Geometry: final body of the model. Coordinates: model frame, mm. Face numbers are marked on the shaded views. A direction names the side the tool comes from. Give positions to 0.01 mm unless a question says otherwise; leave off trailing zeros. Order: outer loops, then holes, each group sorted by start corner. A loop starts at its lowest first (then second) coordinate and runs counter-clockwise, first axis right, second up. Notation, with made-up numbers: (48, 23.25) - (86, 23.25) arc R23 cw to (86, 61.25) - close; hole circle Ø11 at (82, 4.5). An arc over 180 degrees is marked (long way). Use one line per item in the form item = value.
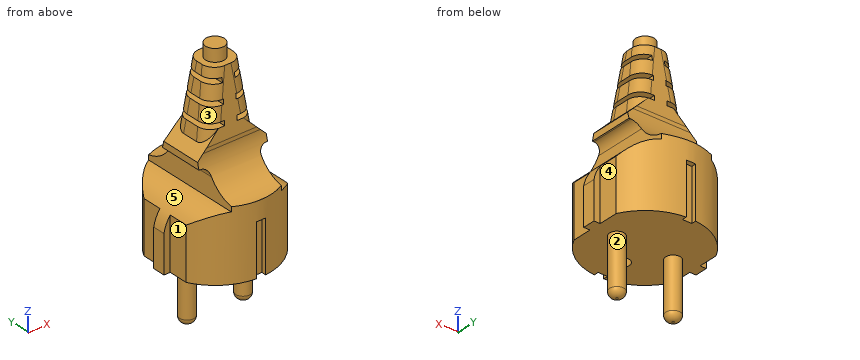
from build123d import *

# Parameters (mm, degrees)
BOSS_EXTRUDE1_DEPTH  = 55.5
SKETCH4_OUTSIDE_W    = 53.062
SKETCH4_OUTSIDE_H    = 72.562
CUT_EXTRUDE3_DEPTH   = 20
CUT_EXTRUDE4_DEPTH   = 16.5
SKETCH6_R            = 5
BOSS_EXTRUDE3_DEPTH  = 55.5
SKETCH7_OUTSIDE_W    = 72.562
SKETCH7_OUTSIDE_H    = 53.062
CUT_EXTRUDE6_DEPTH   = 27.75
FILLET3_R            = 4
SKETCH8_R            = 2.35
BOSS_EXTRUDE4_DEPTH  = 18
FILLET4_R            = 2
FILLET4_OF_MIRROR2_R = 2
SKETCH10_W           = 8.464758564
SKETCH10_H           = 1.5
CUT_EXTRUDE8_DEPTH   = 12
SKETCH11_R           = 3
BOSS_EXTRUDE6_DEPTH  = 59.5
SKETCH12_R           = 2.35
CUT_EXTRUDE9_DEPTH   = 10


with BuildPart() as part:
    # Sketch1 → Boss-Extrude1 (new body)
    with BuildSketch(Plane.XY):
        with BuildLine():
            Line((-16, 2), (-16, 8.246211251))
            ThreePointArc((-16, 8.246211251), (0, 18), (16, 8.246211251))
            Line((16, 8.246211251), (16, 2))
            Line((16, 2), (18, 2))
            Line((18, 2), (18, -2))
            Line((18, -2), (16, -2))
            Line((16, -2), (16, -8.246211251))
            ThreePointArc((16, -8.246211251), (0, -18), (-16, -8.246211251))
            Line((-16, -8.246211251), (-16, -2))
            Line((-16, -2), (-18, -2))
            Line((-18, -2), (-18, 2))
            Line((-18, 2), (-16, 2))
        make_face()
    extrude(amount=BOSS_EXTRUDE1_DEPTH)

    # Sketch4 outside → Cut-Extrude3 (cut, symmetric)
    with BuildSketch(Plane(origin=(0, 0, 0), x_dir=(1, 0, 0), z_dir=(0, 1, 0))):
        with Locations((0, -27.75)):
            Rectangle(SKETCH4_OUTSIDE_W, SKETCH4_OUTSIDE_H)
        with BuildLine():
            Line((-18, 0), (-18, -12))
            ThreePointArc((-18, -12), (-14.536312565, -18.207013961), (-8, -21))
            Line((-8, -21), (-8, -27.5))
            ThreePointArc((-8, -27.5), (-8.732233047, -29.267766953), (-10.5, -30))
            Line((-10.5, -30), (-11, -30))
            Line((-11, -30), (-11, -32))
            Line((-11, -32), (-8, -35))
            Line((-8, -35), (-5, -55.5))
            Line((-5, -55.5), (5, -55.5))
            Line((5, -55.5), (8, -35))
            Line((8, -35), (11, -32))
            Line((11, -32), (11, -30))
            Line((11, -30), (10.5, -30))
            ThreePointArc((10.5, -30), (8.732233047, -29.267766953), (8, -27.5))
            Line((8, -27.5), (8, -21))
            ThreePointArc((8, -21), (14.536312565, -18.207013961), (18, -12))
            Line((18, -12), (18, 0))
            Line((18, 0), (-18, 0))
        make_face(mode=Mode.SUBTRACT)
    extrude(amount=CUT_EXTRUDE3_DEPTH, both=True, mode=Mode.SUBTRACT)

    # Sketch5 → Cut-Extrude4 (cut)
    with BuildSketch(Plane(origin=(0, 0, 0), x_dir=(-1, 0, 0), z_dir=(0, 0, -1))):
        Polygon((0, 19.680001022), (1.5, 19.680001022), (1.5, 17.937391115), (1.5, 16.437391115), (-1.5, 16.437391115), (-1.5, 19.680001022), align=None)
    cut_extrude4 = extrude(amount=-CUT_EXTRUDE4_DEPTH, mode=Mode.SUBTRACT)

    # Mirror1: Cut-Extrude4 across plane
    add(cut_extrude4.mirror(Plane.ZX), mode=Mode.SUBTRACT)

    # Sketch6 → Boss-Extrude3 (add)
    with BuildSketch(Plane.XY):
        Circle(SKETCH6_R)
    extrude(amount=BOSS_EXTRUDE3_DEPTH)

    # Sketch7 outside → Cut-Extrude6 (cut, symmetric)
    with BuildSketch(Plane(origin=(0, 0, 0), x_dir=(0, 0, -1), z_dir=(1, 0, 0))):
        with Locations((-27.75, 0)):
            Rectangle(SKETCH7_OUTSIDE_W, SKETCH7_OUTSIDE_H)
        with BuildLine():
            Line((-22.4, 17.937391115), (-22.4, 20.910001086))
            Line((-22.4, 20.910001086), (0, 20.910001086))
            Line((0, 20.910001086), (0, 17.937391115))
            Line((0, 17.937391115), (0, -17.937391115))
            Line((0, -17.937391115), (0, -20.333967998))
            Line((0, -20.333967998), (-22.4, -20.333967998))
            Line((-22.4, -20.333967998), (-22.4, -17.9))
            ThreePointArc((-22.4, -17.9), (-25.738982694, -9.838982694), (-33.8, -6.5))
            Line((-33.8, -6.5), (-35, -6.5))
            Line((-35, -6.5), (-55.5, -5))
            Line((-55.5, -5), (-55.5, 5))
            Line((-55.5, 5), (-35, 6.5))
            Line((-35, 6.5), (-33.8, 6.5))
            ThreePointArc((-33.8, 6.5), (-25.738982694, 9.838982694), (-22.4, 17.9))
            Line((-22.4, 17.9), (-22.4, 17.937391115))
        make_face(mode=Mode.SUBTRACT)
    extrude(amount=CUT_EXTRUDE6_DEPTH, both=True, mode=Mode.SUBTRACT)

    # Fillet3
    # the kernel refuses this fillet: 4 mm, written as the material it takes off along each edge
    with BuildSketch(Plane(origin=(3.570969245, 4.285484623, 65.26504349), x_dir=(0.010456033399530511, -0.9973894081641158, -0.0714495615632633), z_dir=(0.14442116856011564, 0.07221058427983153, -0.9868779851580924))) as fillet3_piece_1_section:
        with BuildLine():
            CenterArc((FILLET3_R * 0.989488430862, FILLET3_R), FILLET3_R, 180.605445032, 89.394554968)
            Line((-FILLET3_R * 0.0104557388149, FILLET3_R * 0.989433187404), (0, 0))
            Line((0, 0), (FILLET3_R * 0.989488430862, 0))
        make_face()
    fillet3_piece_1 = extrude(amount=40.562346695, mode=Mode.PRIVATE)
    fillet3_piece_1 = split(fillet3_piece_1, bisect_by=Plane(origin=(-1.347793771, 4.447005001, 44.347793771), z_dir=(0.7071067811865519, 0, 0.7071067811865431)), keep=Keep.TOP, mode=Mode.PRIVATE)
    add(fillet3_piece_1, mode=Mode.SUBTRACT)
    with BuildSketch(Plane(origin=(9.429030755, -7.214515377, 25.23495651), x_dir=(0.01045603339953013, 0.9973894081641159, -0.07144956156326311), z_dir=(-0.14442116856011564, 0.07221058427983126, 0.9868779851580924))) as fillet3_piece_2_section:
        with BuildLine():
            CenterArc((FILLET3_R * 0.989488430862, FILLET3_R), FILLET3_R, 180.605445032, 89.394554968)
            Line((-FILLET3_R * 0.0104557388149, FILLET3_R * 0.989433187404), (0, 0))
            Line((0, 0), (FILLET3_R * 0.989488430862, 0))
        make_face()
    fillet3_piece_2 = extrude(amount=40.562346695, mode=Mode.PRIVATE)
    fillet3_piece_2 = split(fillet3_piece_2, bisect_by=Plane(origin=(-1.347793771, -4.447005001, 44.347793771), z_dir=(0.7071067811865519, 0, 0.7071067811865431)), keep=Keep.TOP, mode=Mode.PRIVATE)
    add(fillet3_piece_2, mode=Mode.SUBTRACT)
    with BuildSketch(Plane(origin=(-9.429030755, 7.214515377, 25.23495651), x_dir=(-0.010456033399530862, -0.9973894081641158, -0.07144956156326325), z_dir=(0.14442116856011541, -0.07221058427983153, 0.9868779851580924))) as fillet3_piece_3_section:
        with BuildLine():
            CenterArc((FILLET3_R * 0.989488430862, FILLET3_R), FILLET3_R, 180.605445032, 89.394554968)
            Line((-FILLET3_R * 0.0104557388149, FILLET3_R * 0.989433187404), (0, 0))
            Line((0, 0), (FILLET3_R * 0.989488430862, 0))
        make_face()
    fillet3_piece_3 = extrude(amount=40.562346695, mode=Mode.PRIVATE)
    fillet3_piece_3 = split(fillet3_piece_3, bisect_by=Plane(origin=(1.347793771, 4.447005001, 44.347793771), z_dir=(-0.7071067811865516, 0, 0.7071067811865436)), keep=Keep.TOP, mode=Mode.PRIVATE)
    add(fillet3_piece_3, mode=Mode.SUBTRACT)
    with BuildSketch(Plane(origin=(-3.570969245, -4.285484623, 65.26504349), x_dir=(0.9895163091489351, -0.010539226961374241, -0.1440361018055054), z_dir=(-0.14442116856011541, -0.07221058427983126, -0.9868779851580924))) as fillet3_piece_4_section:
        with BuildLine():
            CenterArc((FILLET3_R * 0.989488430862, -FILLET3_R), FILLET3_R, 90, 89.394554968)
            Line((-FILLET3_R * 0.0104557388149, -FILLET3_R * 0.989433187404), (0, 0))
            Line((0, 0), (FILLET3_R * 0.989488430862, 0))
        make_face()
    fillet3_piece_4 = extrude(amount=40.562346695, mode=Mode.PRIVATE)
    fillet3_piece_4 = split(fillet3_piece_4, bisect_by=Plane(origin=(1.347793771, -4.447005001, 44.347793771), z_dir=(-0.7071067811865516, 0, 0.7071067811865436)), keep=Keep.TOP, mode=Mode.PRIVATE)
    add(fillet3_piece_4, mode=Mode.SUBTRACT)

    # Sketch8 → Boss-Extrude4 (add)
    with BuildSketch(Plane(origin=(0, 0, 0), x_dir=(-1, 0, 0), z_dir=(0, 0, -1))):
        with Locations(Location((-9, 0, 0), (0, 0, 180))):
            Circle(SKETCH8_R)
    boss_extrude4 = extrude(amount=BOSS_EXTRUDE4_DEPTH)

    # Fillet4
    fillet4_edges = [part.edges().sort_by_distance(p)[0] for p in [
        (6.65, 0, -18),
    ]]
    fillet(fillet4_edges, radius=FILLET4_R)

    # Mirror2: Boss-Extrude4 across plane
    add(boss_extrude4.mirror(Plane(origin=(0, 0, 0), x_dir=(0, 0, 1), z_dir=(1, 0, 0))))

    # Fillet4 of Mirror2
    fillet4_of_mirror2_edges = [part.edges().sort_by_distance(p)[0] for p in [
        (-6.65, 0, -18),
    ]]
    fillet(fillet4_of_mirror2_edges, radius=FILLET4_OF_MIRROR2_R)

    # Sketch10 → Cut-Extrude8 (cut, symmetric)
    with BuildSketch(Plane(origin=(0, 0, 0), x_dir=(1, 0, 0), z_dir=(0, 1, 0))):
        with Locations((6.232463803, -39.75)):
            Rectangle(SKETCH10_W, SKETCH10_H)
        with Locations((6.232463803, -45.75)):
            Rectangle(SKETCH10_W, SKETCH10_H)
        with Locations((6.232463803, -51.75)):
            Rectangle(SKETCH10_W, SKETCH10_H)
        with Locations((-6.232463803, -51.75)):
            Rectangle(SKETCH10_W, SKETCH10_H)
        with Locations((-6.232463803, -45.75)):
            Rectangle(SKETCH10_W, SKETCH10_H)
        with Locations((-6.232463803, -39.75)):
            Rectangle(SKETCH10_W, SKETCH10_H)
    extrude(amount=CUT_EXTRUDE8_DEPTH, both=True, mode=Mode.SUBTRACT)

    # Sketch11 → Boss-Extrude6 (add)
    with BuildSketch(Plane.XY):
        Circle(SKETCH11_R)
    extrude(amount=BOSS_EXTRUDE6_DEPTH)

    # Sketch12 → Cut-Extrude9 (cut)
    with BuildSketch(Plane(origin=(0, 0, 0), x_dir=(-1, 0, 0), z_dir=(0, 0, -1))):
        with Locations((0, -9)):
            Circle(SKETCH12_R)
    extrude(amount=-CUT_EXTRUDE9_DEPTH, mode=Mode.SUBTRACT)


solid = part.part
(1) Cut plane D-D on z = 33. Output: boundary loops of the cut face in (x, y).
Computed values:
outline = (-10, -6.53) - (10, -6.53) - (10, 6.53) - (-10, 6.53) - close
(2) Cut plane B-B on x = 0. Output: boundary loops of the cut face in (y, z), plus the area to 3 significant figures.
Computed values:
outline = (-18, 16.5) - (-16.44, 16.5) - (-16.44, 0) - (-11.35, 0) - (-11.35, 10) - (-6.65, 10) - (-6.65, 0) - (16.44, 0) - (16.44, 16.5) - (18, 16.5) - (18, 22.4) - (17.9, 22.4) arc R11.4 cw to (6.5, 33.8) - (6.5, 35) - (5, 55.5) - (3, 55.5) - (3, 59.5) - (-3, 59.5) - (-3, 55.5) - (-5, 55.5) - (-6.5, 35) - (-6.5, 33.8) arc R11.4 cw to (-17.9, 22.4) - (-18, 22.4) - close
area = 1,190 mm²
(3) Reachability of the marked faces 1, 2, 3, 4 and 5 from +Z, -Z, +X, -X, +Y, -Y: full face, straight path, thin tool, end or side. Return the list, or none.
Computed values:
face_1 = +Z, -Z, -X, -Y
face_2 = -Z
face_3 = +Z, -X, -Y
face_4 = +Z, -Z, +X, +Y
face_5 = -X, +Y, -Y
(4) Contact query for flat-ended pins moving along their axis: pin 1 Ø6 at (y, z) = (8, 36.5) entering from +X; pin 2 Ø4.5 at (x, y) = (-4, -2) entering from -Z; pin 3 Ø0.9 at (x, z) = (0.5, 4.5) entering from +Y; pin 4 Ø10 at (y, z) = (-14, 47.5) entering from -X. Output: stop coordinate, or through.
Computed values:
pin_1 = 9.1
pin_2 = 0
pin_3 = 16.44
pin_4 = through
(5) Ray query, line 1 along Y through (x, z) = (0, 7); line 2 along Z through (x, y) = (-5, 9); line 3 along Z through (x, y) = (12.5, -5.5). Return the intervals inside material, ascending.
Computed values:
line_1 = -16.44 to -11.35, -6.65 to 16.44
line_2 = 0 to 26.68
line_3 = 0 to 19.66
(6) Cut plane A-A on z = 8.5. Output: boundary loops of the cut face in (x, y), plus the area to 3 significant figures.
Computed values:
outline = (-18, -2) - (-16, -2) - (-16, -8.25) arc R18 ccw to (-1.5, -17.94) - (-1.5, -16.44) - (1.5, -16.44) - (1.5, -17.94) arc R18 ccw to (16, -8.25) - (16, -2) - (18, -2) - (18, 2) - (16, 2) - (16, 8.25) arc R18 ccw to (1.5, 17.94) - (1.5, 16.44) - (-1.5, 16.44) - (-1.5, 17.94) arc R18 ccw to (-16, 8.25) - (-16, 2) - (-18, 2) - close; hole circle Ø4.7 at (0, -9)
area = 963 mm²
(7) Cut plane C-C on z = -2. Output: boundary loops of the cut face in (x, y), plus the area to 3 significant figures.
Computed values:
outline = circle Ø4.7 at (-9, 0); circle Ø4.7 at (9, 0)
area = 34.7 mm²
